The listing builds one solid part. Answer for the finished solid, in the listing's coordinates (mm). A direction names the side the tool comes from. Give positions to 0.01 mm unless a question says otherwise; leave off trailing zeros. Write each loop counter-clockwise with the first axis right and the second up, starting at its lowest first coordinate (ties: lowest second). Pieces come first, ordered by that corner, then holes.
```python
from build123d import *

# Parameters (mm, degrees)
SKETCH2_R           = 10
SKETCH2_R_2         = 1
BOSS_EXTRUDE2_DEPTH = 9
CUT_EXTRUDE4_DEPTH  = 10
CIRPATTERN2_COUNT   = 11
SKETCH7_R           = 2
SKETCH7_R_2         = 1
CUT_EXTRUDE5_DEPTH  = 7.5


with BuildPart() as part:
    # Sketch2 → Boss-Extrude2 (new body)
    with BuildSketch(Plane(origin=(0, 0, 0), x_dir=(0, 0, -1), z_dir=(1, 0, 0))):
        Circle(SKETCH2_R)
        Circle(SKETCH2_R_2, mode=Mode.SUBTRACT)
    extrude(amount=BOSS_EXTRUDE2_DEPTH)

    # Sketch6 → Cut-Extrude4 (cut, symmetric)
    with BuildSketch(Plane(origin=(0, 0, 0), x_dir=(0, 0, -1), z_dir=(1, 0, 0))):
        with BuildLine():
            ThreePointArc((1.85, 9.889708377), (0, 10.025881913), (-1.85, 9.889708377))
            add(Edge.make_bspline(
                [(-0.85, 7.986983034), (-1.133345999, 8.672201219), (-1.446471777, 9.32650192), (-1.85, 9.889708377)],
                knots=[0.309355195, 0.309355195, 0.309355195, 0.309355195, 0.515063523, 0.515063523, 0.515063523, 0.515063523], degree=3))
            ThreePointArc((-0.85, 7.986983034), (0, 8.021021821), (0.85, 7.986983034))
            add(Edge.make_bspline(
                [(0.85, 7.986983034), (1.133345999, 8.672201219), (1.446471777, 9.32650192), (1.85, 9.889708377)],
                knots=[0.309355195, 0.309355195, 0.309355195, 0.309355195, 0.515063523, 0.515063523, 0.515063523, 0.515063523], degree=3))
        make_face()
    cut_extrude4 = extrude(amount=CUT_EXTRUDE4_DEPTH, both=True, mode=Mode.SUBTRACT)

    # CirPattern2: Cut-Extrude4 ×11 about axis
    cirpattern2_axis = Axis((9, 0, 0), (-1, 0, 0))
    for i in range(1, CIRPATTERN2_COUNT):
        add(cut_extrude4.rotate(cirpattern2_axis, i * 360 / CIRPATTERN2_COUNT), mode=Mode.SUBTRACT)

    # Sketch7 → Cut-Extrude5 (cut)
    with BuildSketch(Plane(origin=(9, 0, 0), x_dir=(0, 0, -1), z_dir=(1, 0, 0))):
        Circle(SKETCH7_R)
        Circle(SKETCH7_R_2, mode=Mode.SUBTRACT)
    extrude(amount=-CUT_EXTRUDE5_DEPTH, mode=Mode.SUBTRACT)


solid = part.part
```
Item 1: Which of the six approach directions +Z, -Z, +X, -X, +Y, -Y give full straight-line access (tool end or side, diameter ignored) to faces 1 (the face through (4.56, -1.15, 7.94)), 2 (the face through (4.44, -4.17, -9.09)), 3 (the face through (4.563, -5.244, -6.07)), 4 (the face through (5, -2, 0)), 5 (the face through (4.56, -7.7, 2.25))?
Conclusion:
face 1: +Z, +X, -X
face 2: -Z, +X, -X, -Y
face 3: +X, -X
face 4: +X
face 5: +X, -X, -Y
Item 2: Consider probe 1 along Y at (x, z) = (0.45, 0); probe 2 along Y at (x, z) = (3.25, 0); probe 3 along Z at (x, y) = (2.25, -8). Determine where each line is inside the solid, lowest interval first.
Conclusion:
probe 1: y = -10 to -1, 1 to 8.02
probe 2: y = -10 to -2, 2 to 8.02
probe 3: z = -6 to -3.55, -1.42 to 1.42, 3.55 to 6
Item 3: Determine the mould class of faces 6 (the face through (4.56, 6.74, 4.35)), 7 (the face through (4.437, -8.405, 5.419)), 8 (the face through (4.4, 6.5, -7.6)) for opening direction Z: pulls with the +Z half, pulls with the -Z half, needs draft (parallel to the pull), parting line crosses it, or undercut.
Conclusion:
face 6: undercut
face 7: pulls with the +Z half
face 8: pulls with the -Z half
Item 4: Each of these flat-tipped pins is pushed along its axis until it touches: P1, Ø1.5, axis at x = 2, y = -1.5, coming from the -Z side; P2, Ø3, axis at x = 5, z = -6.5, coming from the -Y side; P3, Ø2, axis at x = 2, z = -3, coming from the -Y side. Where does it stop, or does it pass through?
Conclusion:
P1: stops at z = -8.23
P2: stops at y = -8.66
P3: stops at y = -8.47
Item 5: A cutting plane is placed at B-B, the plane y = 0.75. Give the vertices of the cut face in (x, z).
Conclusion:
outline: (0, -9.97) - (9, -9.97) - (9, -1.85) - (1.5, -1.85) - (1.5, -0.66) - (0, -0.66) - close; (0, 0.66) - (1.5, 0.66) - (1.5, 1.85) - (9, 1.85) - (9, 9.97) - (0, 9.97) - close
Item 6: A cutting plane is placed at A-A, the plane z = 0. Give the vertices of the cut face in (x, y).
Conclusion:
outline: (0, -10) - (9, -10) - (9, -2) - (1.5, -2) - (1.5, -1) - (0, -1) - close; (0, 1) - (1.5, 1) - (1.5, 2) - (9, 2) - (9, 8.02) - (0, 8.02) - close
